The figure shows three views and two pictorial views of one solid part (mm, origin at its lowest corner). Answer the questions. Round coordinates to 2 decimals unless told otherwise and drop trailing zeros. Order: outer loops, then holes, each group sorted by start corner. A loop starts at its lowest first (then second) coordinate and runs counter-clockwise, first axis right, second up. Notation, with made-up numbers: (12.25, 44.5) - (40.25, 44.5) arc R32 cw to (40.25, 72.5) - close; hole circle Ø5 at (74.5, -12). An arc over 180 degrees is marked (long way). Answer in a Markdown table with one row per item.
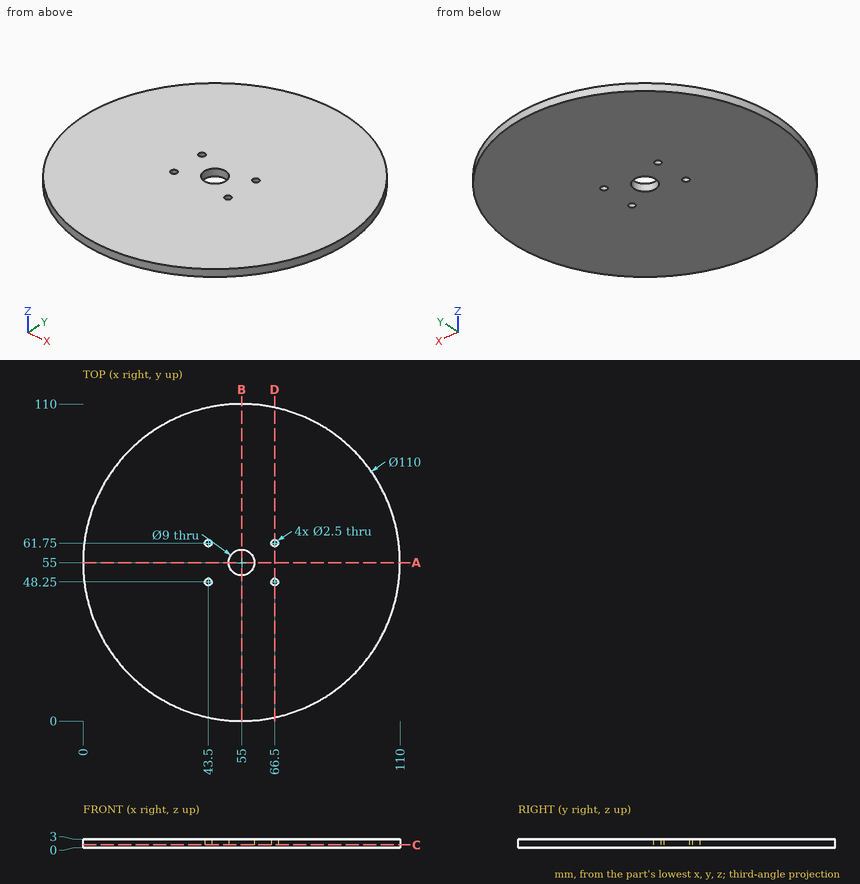
1) Find the intervals of material crossed by probe 1 along Y at (x, z) = (55, 1.1); probe 2 along X at (y, z) = (61.75, 0.6); probe 3 along Y at (x, z) = (43.5, 2.2), in increasing order. Write a range as from..to.
Filled in:
| item | result |
|---|---|
| probe 1 | y = 0..50.5, 59.5..110 |
| probe 2 | x = 0.42..42.25, 44.75..65.25, 67.75..109.58 |
| probe 3 | y = 1.22..47, 49.5..60.5, 63..108.78 |
2) Find section D-D, the plane x = 66.5. Give the vertices of the cut face in (y, z), then the cut area to 3 significant figures.
Filled in:
| item | result |
|---|---|
| outline | (1.22, 0) - (47, 0) - (47, 3) - (1.22, 3) - close; (49.5, 0) - (60.5, 0) - (60.5, 3) - (49.5, 3) - close; (63, 0) - (108.78, 0) - (108.78, 3) - (63, 3) - close |
| area | 308 mm^2 |
3) Each of these flat-tipped pins is pushed along its axis until it touches: pin 1 (1 mm diameter, centred on y = 83.5, z = 2.5, fed in from -X); pin 2 (1 mm diameter, centred on y = 12.5, z = 2, fed in from -X); pin 3 (1.5 mm diameter, centred on x = 30.5, z = 2, fed in from +Y). Where does it stop, or does it pass through?
Filled in:
| item | result |
|---|---|
| pin 1 | stops at x = 7.66 |
| pin 2 | stops at x = 19.49 |
| pin 3 | stops at y = 104.61 |
4) Find section C-C, the plane z = 1. Give the vertices of the cut face in (x, y).
Filled in:
| item | result |
|---|---|
| outline | circle Ø110 at (55, 55); hole circle Ø2.5 at (43.5, 48.25); hole circle Ø2.5 at (43.5, 61.75); hole circle Ø9 at (55, 55); hole circle Ø2.5 at (66.5, 48.25); hole circle Ø2.5 at (66.5, 61.75) |
5) Find section A-A, the plane y = 55. Give the vertices of the cut face in (x, z), then the cut area to 3 significant figures.
Filled in:
| item | result |
|---|---|
| outline | (0, 0) - (50.5, 0) - (50.5, 3) - (0, 3) - close; (59.5, 0) - (110, 0) - (110, 3) - (59.5, 3) - close |
| area | 303 mm^2 |
